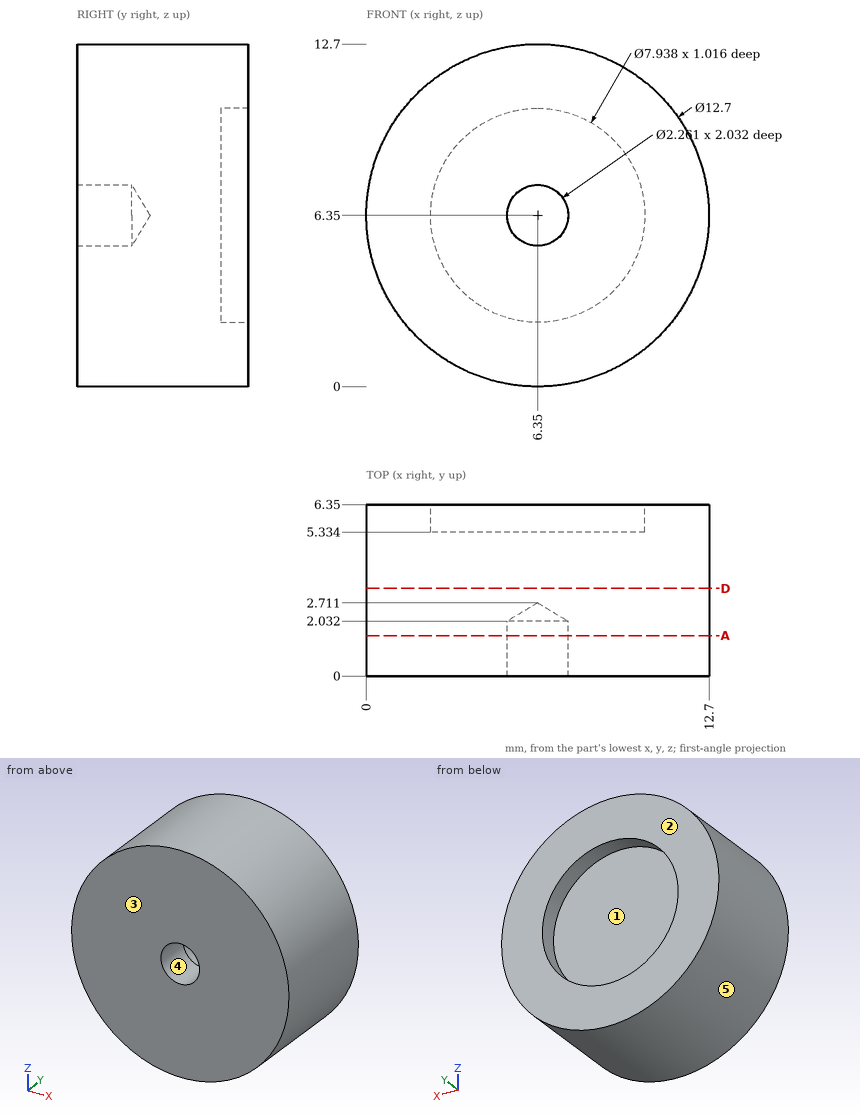
The figure shows three views and two pictorial views of one solid part (mm, origin at its lowest corner). Answer the questions. A direction names the side the tool comes from. Coordinates: 2 decimals unless noted, no trailing zeros. Loops run counter-clockwise (first coordinate to the right, second up) from the corner with the lowest first, then second, coordinate; pieces in that order, holes last. Notation, with made-up numbers: (40, -28.5) -> (72, -28.5) arc R19 cw to (72, 0.5) -> close; hole circle Ø11 at (5.5, 22). An arc over 180 degrees is marked (long way). Return JSON: item names as keys, results as strings. Group by question number.
(1) Determine the mould class of the marked faces 3, 4 and 5 for opening direction Z: released by +Z, released by -Z, zero draft, split by the parting line, or undercut.
(2) A cutting plane is placed at D-D on y = 3.25. Write down the section's boundary in (x, z), and give its area (3 significant figures).
(3) Given pin 1 Ø5 at (x, z) = (6.35, 6.35) entering from +Y; pin 2 Ø1.5 at (x, y) = (2.5, 2) entering from +Z, each flat-ended and moving along its own axis, determine where each tip first touches the part or whether it passes through.
(4) Which of the six approach directions +Z, -Z, +X, -X, +Y, -Y give full straight-line access (tool end or side, diameter ignored) to the marked faces 1 and 2?
(5) A cutting plane is placed at A-A on y = 1.5. Write down the section's boundary in (x, z).
(6) Find the intervals of material crossed by probe 1 along X at (y, z) = (1.25, 6.35); probe 2 along X at (y, z) = (5.6, 6.35); probe 3 along Y at (x, z) = (9, 5.5) (1 decimal), in increasing order. Write a range as from..to.
The answers:
{
 "1": {"face 3": "zero draft", "face 4": "undercut", "face 5": "split by the parting line"},
 "2": {"outline": "circle Ø12.7 at (6.35, 6.35)", "area": "127 mm^2"},
 "3": {"pin 1": "stops at y = 5.33", "pin 2": "stops at z = 11.89"},
 "4": {"face 1": "+Y", "face 2": "+Z, -Z, +X, -X, +Y"},
 "5": {"outline": "circle Ø12.7 at (6.35, 6.35); hole circle Ø2.26 at (6.35, 6.35)"},
 "6": {"probe 1": "x = 0..5.22, 7.48..12.7", "probe 2": "x = 0..2.38, 10.32..12.7", "probe 3": "y = 0..5.3"}
}
